```python
from build123d import *


with BuildPart() as part:
    # Sketch1 → Revolve1 (revolve)
    with BuildSketch(Plane.XY):
        with BuildLine():
            Line((0, 0), (0, 70.258458908))
            add(Edge.make_bspline(
                [(0, 70.258458908), (3.42486489, 70.528708067), (6.542490016, 68.711522876)],
                knots=[0, 0, 0, 1, 1, 1], degree=2))
            Line((6.542490016, 68.711522876), (2.569010768, 68.711522876))
            Line((2.569010768, 68.711522876), (2.569010768, 44.624031208))
            Line((2.569010768, 44.624031208), (10.316772859, 44.624031208))
            add(Edge.make_bspline(
                [(10.316772859, 44.624031208), (12.045144659, 44.645198788), (12.886059681, 43.724390653)],
                knots=[0, 0, 0, 1, 1, 1], degree=2))
            Line((12.886059681, 43.724390653), (0.749314242, 43.724390653))
            Line((0.749314242, 43.724390653), (0.193971896, 1.407170555))
            Line((0.193971896, 1.407170555), (0, 0))
        make_face()
    revolve(axis=Axis((0, 0, 0), (0, 1, 0)))


solid = part.part
```
Could you check a few things on this model? Use its own coordinates, in mm. Round coordinates to 2 decimals unless told otherwise and drop trailing zeros. Write each loop counter-clockwise with the first axis right and the second up, starting at its lowest first coordinate (ties: lowest second). Pieces come first, ordered by that corner, then holes. Notation, with made-up numbers: M -12,52 L 20,52 A24 cw 20,67 Z; hole C -11,-39.75 d7. An arc over 180 degrees is marked long. Write each question's results on one line, items separated by ' | '. Start each with the question number.
1. Imagine slicing it at B-B on y = 11. List the corners of the cut face in (x, z) for me, and give its area (3 significant figures).
2. I need wall thicknesses on L1, parallel to Y at x = -5.25, z = 1; L2, parallel to Y at x = -1.25, z = 5.5; L3, parallel to Y at x = -8, z = 5. Which ranges of each line are inside material? Lowest first, please. Write a range as from..to.
3. Imagine slicing it at A-A on y = 35.5. List the corners of the cut face in (x, z) for me.
4. I'm going to push flat-ended pins straight in: pin 1 Ø7.5 at (x, z) = (5.5, 4.5) entering from -Y; pin 2 Ø6 at (y, z) = (33.5, -5) entering from -X; pin 3 Ø8 at (x, z) = (-3, -6) entering from +Y; pin 4 Ø8 at (x, y) = (0.5, 53) entering from +Z. Where does each tip first touch, or does it pass through?
5. Thinking about a two-plate mould opening in Y: for faces 1 (the face through (0.446, 22.27, -0.141)), 2 (the face through (3, 68.712, 0)), 3 (the face through (-2, 44.624, 2)), which applies, +Y half, -Y half, draft (parallel to the pull), parting line (faces both ways), or undercut?
Result sheet:
1) outline: C 0,0 d0.64 | area: 0.321 mm^2
2) L1: y = 43.72..44.62, 68.71..69.33 | L2: y = 43.72..44.62, 68.71..69.19 | L3: y = 43.72..44.62
3) outline: C 0,0 d1.28
4) pin 1: stops at y = 43.72 | pin 2: passes through | pin 3: stops at y = 70.14 | pin 4: stops at z = 2.57
5) face 1: -Y half | face 2: undercut | face 3: undercut
